Work out the finished part from the listing and answer in its coordinate system (mm). A direction names the side the tool comes from. Coordinates: 2 decimals unless noted, no trailing zeros. Order: outer loops, then holes, each group sorted by start corner. A loop starts at its lowest first (then second) coordinate and runs counter-clockwise, first axis right, second up. Notation, with made-up numbers: (58.25, 88) -> (74.25, 88) arc R24 cw to (74.25, 109) -> close; hole circle Ø3 at (74, 78.25). An arc over 180 degrees is marked (long way). Use one line per item in the form item = value.
from build123d import *

# Parameters (mm, degrees)
F1_DEPTH = 9.652
F3_R     = 3.175
F4_DEPTH = 55.88
F5_W     = 19.1262
F5_H     = 2.54
F5_H_2   = 1.292995
F6_DEPTH = 25.4


with BuildPart() as f1:
    # F0 (on Front) → F1 (new body)
    with BuildSketch(Plane.XZ):
        Polygon((-44.798229, 15.301452), (-44.798229, 40.701452), (-50.881937, 40.701452), (-50.881937, 6.821129), (-25.748229, 6.821129), (-25.748229, -10.098548), (-19.398229, -10.098548), (-19.398229, 15.301452), align=None)
    extrude(amount=F1_DEPTH)

    # F3 (on Right) → F4 (cut)
    with BuildSketch(Plane.YZ):
        with Locations((-4.7498, 31.888157)):
            Circle(F3_R)
    extrude(amount=-F4_DEPTH, mode=Mode.SUBTRACT)

    # F5 (on Front) → F6 (cut)
    with BuildSketch(Plane.XZ):
        with Locations((-35.158537, 12.950574)):
            Rectangle(F5_W, F5_H)
        with Locations((-35.158537, 14.867071)):
            Rectangle(F5_W, F5_H_2)
    extrude(amount=F6_DEPTH, mode=Mode.SUBTRACT)


solid = f1.part
(1) Straight lines are drawn through the part: line 1 along X through (y, z) = (-7.5, 14.5); line 2 along X through (y, z) = (-6.75, -7.5); line 3 along Z through (x, y) = (-25, -7.25). For each, find the intervals that lie inside material, in ascending order.
Data:
line_1 = -50.88 to -44.72, -25.6 to -19.4
line_2 = -25.75 to -19.4
line_3 = -10.1 to 15.3
(2) Section B-B on z = 30 is taken. Write down the section's boundary in (x, y).
Data:
outline = (-50.88, -9.65) -> (-44.8, -9.65) -> (-44.8, -7.3) -> (-50.88, -7.3) -> close; (-50.88, -2.2) -> (-44.8, -2.2) -> (-44.8, 0) -> (-50.88, 0) -> close
(3) Each of these flat-tipped pins is pushed along its axis until it touches: P1, Ø3, axis at x = -47, y = -2, coming from the -Z side; P2, Ø1.9, axis at x = -22.5, y = -7, coming from the +Z side; P3, Ø3, axis at x = -36.5, y = -3.5, coming from the +Z side. Where does it stop, or does it pass through?
Data:
P1 = 6.82
P2 = 15.3
P3 = 11.68
(4) The mould has two halves that part along X. Classify faces 5 (the flat face through (-23, -5, -10.099)), 6 (the flat face through (-25.595, -5, 13)), 7 (the flat face through (-19.398, -5, 2)): released by +X, released by -X, zero draft, split by the parting line, or undercut.
Data:
face_5 = zero draft
face_6 = undercut
face_7 = released by +X
(5) Section C-C on y = -0.75 is taken. Write down the section's boundary in (x, z), plus the area to 3 significant figures.
Data:
outline = (-50.88, 6.82) -> (-25.75, 6.82) -> (-25.75, -10.1) -> (-19.4, -10.1) -> (-19.4, 15.3) -> (-25.6, 15.3) -> (-25.6, 11.68) -> (-44.72, 11.68) -> (-44.72, 15.3) -> (-44.8, 15.3) -> (-44.8, 40.7) -> (-50.88, 40.7) -> close
area = 460 mm²
(6) Section D-D on x = -28.5 is taken. Write down the section's boundary in (y, z), plus the area to 3 significant figures.
Data:
outline = (-9.65, 6.82) -> (0, 6.82) -> (0, 11.68) -> (-9.65, 11.68) -> close
area = 46.9 mm²
(7) Section A-A on y = -6.75 is taken. Write down the section's boundary in (x, z).
Data:
outline = (-50.88, 6.82) -> (-25.75, 6.82) -> (-25.75, -10.1) -> (-19.4, -10.1) -> (-19.4, 15.3) -> (-25.6, 15.3) -> (-25.6, 11.68) -> (-44.72, 11.68) -> (-44.72, 15.3) -> (-44.8, 15.3) -> (-44.8, 29.42) -> (-50.88, 29.42) -> close; (-50.88, 34.35) -> (-44.8, 34.35) -> (-44.8, 40.7) -> (-50.88, 40.7) -> close
(8) Which of the six approach directions +Z, -Z, +X, -X, +Y, -Y give full straight-line access (tool end or side, diameter ignored) to faces 1 (the flat face through (-44.798, -5, 28)), 2 (the flat face through (-44.722, -5, 14)), 3 (the flat face through (-25.748, -5, -2)), 4 (the flat face through (-48, -5, 40.701))?
Data:
face_1 = +Z, +X, +Y, -Y
face_2 = +Z, +Y, -Y
face_3 = -Z, -X, +Y, -Y
face_4 = +Z, +X, -X, +Y, -Y
